Input: part model. Units: mm. Frame: model coordinates. Round coordinates to 2 decimals unless told otherwise and drop trailing zeros. Loops run counter-clockwise (first coordinate to the right, second up) from the corner with the lowest first, then second, coordinate; pieces in that order, holes last. Notation, with made-up numbers: (37.25, -9) -> (51.25, -9) arc R9 ccw to (51.25, -5) -> close; hole circle Ø3 at (12, 45). An arc over 180 degrees is marked (long way). Answer as a JSON object with one key per item and string values.
```python
from build123d import *

# Parameters (mm, degrees)
SKETCH_1_R          = 2.5
EXTRUDE_1_DEPTH     = 10
SKETCH_2_R          = 0.25
EXTRUDE_2_DEPTH     = 2
SKETCH_3_W          = 1.167779505
SKETCH_3_H          = 0.556477286
CUT_EXTRUDE_1_DEPTH = 0.25


with BuildPart() as part:
    # 草图1 → 凸台-拉伸1 (new body)
    with BuildSketch(Plane.XY):
        Circle(SKETCH_1_R)
    extrude(amount=EXTRUDE_1_DEPTH)

    # 草图2 → 凸台-拉伸2 (add)
    with BuildSketch(Plane(origin=(0, 0, 0), x_dir=(-1, 0, 0), z_dir=(0, 0, -1))):
        with Locations(Location((-1.5, 0, 0), (0, 0, 180))):
            Circle(SKETCH_2_R)
        with Locations(Location((1.5, 0, 0), (0, 0, 180))):
            Circle(SKETCH_2_R)
    extrude(amount=EXTRUDE_2_DEPTH)

    # 草图3 → 切除-拉伸1 (cut)
    with BuildSketch(Plane(origin=(2.5, 0, 0), x_dir=(0, 0, -1), z_dir=(1, 0, 0))):
        with Locations((-8.875568116, 0)):
            Rectangle(SKETCH_3_W, SKETCH_3_H)
        with Locations((-6.875568116, 0)):
            Rectangle(SKETCH_3_W, SKETCH_3_H)
        with Locations((-4.875568116, 0)):
            Rectangle(SKETCH_3_W, SKETCH_3_H)
        with Locations((-2.875568116, 0)):
            Rectangle(SKETCH_3_W, SKETCH_3_H)
        with Locations((-0.875568116, 0)):
            Rectangle(SKETCH_3_W, SKETCH_3_H)
    extrude(amount=-CUT_EXTRUDE_1_DEPTH, mode=Mode.SUBTRACT)


solid = part.part
```
1) Contact query for a flat-ended pin moving along its axis: P1, Ø2, axis at y = -1.5, z = 5.5, coming from the +X side. Output: stop coordinate, or through.
Output:
{"P1": "stops at x = 2.45"}
2) Section B-B, the plane z = -0.25. Output: boundary loops of the cut face in (x, y), plus the area to 3 significant figures.
Output:
{"outline": "circle Ø0.5 at (-1.5, 0); circle Ø0.5 at (1.5, 0)", "area": "0.393 mm^2"}
3) Section D-D, the plane x = 0. Output: boundary loops of the cut face in (y, z), plus the area to 3 significant figures.
Output:
{"outline": "(-2.5, 0) -> (2.5, 0) -> (2.5, 10) -> (-2.5, 10) -> close", "area": "50.0 mm^2"}
4) Section A-A, the plane x = -1.5. Output: boundary loops of the cut face in (y, z), plus the area to 3 significant figures.
Output:
{"outline": "(-2, 0) -> (-0.25, 0) -> (-0.25, -2) -> (0.25, -2) -> (0.25, 0) -> (2, 0) -> (2, 10) -> (-2, 10) -> close", "area": "41.0 mm^2"}
5) Ray query, probe 1 along Z at (x, y) = (0.25, -0.05); probe 2 along Y at (x, z) = (-0.1, 0.5); probe 3 along X at (y, z) = (-0.85, 6.25). Return the intervals inside material, ascending.
Output:
{"probe 1": "z = 0 to 10", "probe 2": "y = -2.5 to 2.5", "probe 3": "x = -2.35 to 2.35"}
